Here's how the part is built. I have some questions about the finished solid (model axes, mm). Coordinates: 2 decimals unless noted, no trailing zeros. Loops run counter-clockwise (first coordinate to the right, second up) from the corner with the lowest first, then second, coordinate; pieces in that order, holes last. Notation, with made-up numbers: (-38.75, 79.5) -> (-9.75, 79.5) arc R6 ccw to (-9.75, 87.5) -> close; hole circle Ø2 at (4, -17). An arc over 180 degrees is marked (long way). Answer as a JSON object with one key per item and string values. Group by question number.
1) I want a section at B-B (x = -19.05). Write out the boundary of the cut face in (y, z), then the cut area to 3 significant figures.
2) I need wall thicknesses on probe 1 along Y at (x, z) = (-253, 1.5); probe 2 along X at (y, z) = (103, 1.5); probe 3 along X at (y, z) = (127.5, 3.75). Which ranges of each line are inside material? Lowest first, please. Write a range as [from, to].
3) I'm going to push flat-ended pins straight in: pin 1 (1.5 mm diameter, centred on y = 40.5, z = 4, fed in from -X); pin 2 (4 mm diameter, centred on x = -107, z = 1.5, fed in from -Y); pin 3 (3 mm diameter, centred on x = -216.5, z = 4, fed in from -Y). Where does each tip first touch, or does it pass through?
4) I want a section at D-D (y = 36). Write out the boundary of the cut face in (x, z), then the cut area to 3 significant figures.
5) I want a section at C-C (x = -192.5). Write out the boundary of the cut face in (y, z).
6) I want a section at A-A (y = 143). Write out the boundary of the cut face in (x, z).
```python
from build123d import *

# Parameters (mm, degrees)
SKETCH2_R               = 28.575
SKETCH2_R_2             = 3.2639
SKETCH2_R_3             = 52.3875
BOSS_EXTRUDE1_DEPTH     = 7.62
CUT_EXTRUDE1_DEPTH      = 369.573342704
CUT_EXTRUDE1_DEPTH_BACK = 369.573342704
SKETCH3_R               = 4.15
SKETCH3_R_2             = 2.5
CUT_EXTRUDE2_DEPTH      = 369.573342704
CUT_EXTRUDE2_DEPTH_BACK = 369.573342704


with BuildPart() as part:
    # Sketch2 → Boss-Extrude1 (new body)
    with BuildSketch(Plane.XY):
        with BuildLine():
            Line((-308.866129262, 91.710399516), (-215.926365234, 14.107506231))
            ThreePointArc((-215.926365234, 14.107506231), (-212.572921228, 12.657721799), (-208.970475069, 13.265869211))
            Line((-208.970475069, 13.265869211), (-134.814952137, 49.535152614))
            ThreePointArc((-134.814952137, 49.535152614), (-114.3, 46.0375), (-93.785047863, 49.535152614))
            Line((-93.785047863, 49.535152614), (-21.949808906, 13.301039962))
            ThreePointArc((-21.949808906, 13.301039962), (-14.699565425, 14.303090245), (-13.070560605, 21.438668609))
            Line((-13.070560605, 21.438668609), (-56.805390428, 130.917967399))
            ThreePointArc((-56.805390428, 130.917967399), (-79.09759936, 158.880822155), (-113.13445351, 169.85152791))
            Line((-113.13445351, 169.85152791), (-257.123397092, 172.562701825))
            ThreePointArc((-257.123397092, 172.562701825), (-258.950279318, 171.836030325), (-259.711214384, 170.023151962))
            Line((-259.711214384, 170.023151962), (-259.711214384, 163.648011794))
            ThreePointArc((-259.711214384, 163.648011794), (-266.061214384, 157.298011794), (-272.411214384, 163.648011794))
            Line((-272.411214384, 163.648011794), (-272.411214384, 170.357932335))
            ThreePointArc((-272.411214384, 170.357932335), (-273.138336021, 172.136997269), (-274.903397092, 172.897482198))
            Line((-274.903397092, 172.897482198), (-278.534507017, 172.96585252))
            ThreePointArc((-278.534507017, 172.96585252), (-281.325275441, 172.933669465), (-284.108948518, 172.732203969))
            ThreePointArc((-284.108948518, 172.732203969), (-285.734576401, 171.907148337), (-286.388785616, 170.205562866))
            Line((-286.388785616, 170.205562866), (-286.388785616, 163.648011794))
            ThreePointArc((-286.388785616, 163.648011794), (-292.738785616, 157.298011794), (-299.088785616, 163.648011794))
            Line((-299.088785616, 163.648011794), (-299.088785616, 164.31478857))
            ThreePointArc((-299.088785616, 164.31478857), (-300.373839326, 166.523115948), (-302.928714599, 166.496939949))
            ThreePointArc((-302.928714599, 166.496939949), (-325.229794091, 130.638495508), (-308.866129262, 91.710399516))
        make_face()
        with Locations(Location((-279.4, 127, 0), (0, 0, 180))):
            Circle(SKETCH2_R, mode=Mode.SUBTRACT)
        with Locations(Location((-19.05, 19.05, 0), (0, 0, 180))):
            Circle(SKETCH2_R_2, mode=Mode.SUBTRACT)
        with Locations(Location((-211.799479175, 19.05, 0), (0, 0, 180))):
            Circle(SKETCH2_R_2, mode=Mode.SUBTRACT)
        with Locations(Location((-114.3, 107.95, 0), (0, 0, 180))):
            Circle(SKETCH2_R_3, mode=Mode.SUBTRACT)
    extrude(amount=BOSS_EXTRUDE1_DEPTH)

    # Sketch3 → Cut-Extrude1 (cut, two sides: drawn at the far end of the back side and taken through both)
    with BuildSketch(Plane.XY.offset(7.62).offset(-CUT_EXTRUDE1_DEPTH_BACK)):
        with Locations((-279.4, 166.00043)):
            Circle(SKETCH3_R)
        with Locations((-254.746524018, 156.380868571)):
            Circle(SKETCH3_R)
        with Locations((-242.044200635, 133.164908097)):
            Circle(SKETCH3_R)
        with Locations((-247.236588134, 107.215554499)):
            Circle(SKETCH3_R)
        with Locations((-267.894110695, 90.674798722)):
            Circle(SKETCH3_R)
        with Locations((-294.35088393, 91.282244222)):
            Circle(SKETCH3_R)
        with Locations((-314.227489609, 108.753660501)):
            Circle(SKETCH3_R)
        with Locations((-318.223443029, 134.913977707)):
            Circle(SKETCH3_R)
        with Locations((-304.468993176, 157.522492681)):
            Circle(SKETCH3_R)
        with Locations((-114.3, 165.1)):
            Circle(SKETCH3_R_2)
        with Locations((-80.708072831, 154.185321229)):
            Circle(SKETCH3_R_2)
        with Locations((-59.947120094, 125.610321229)):
            Circle(SKETCH3_R_2)
        with Locations((-59.947120094, 90.289678771)):
            Circle(SKETCH3_R_2)
        with Locations((-80.708072831, 61.714678771)):
            Circle(SKETCH3_R_2)
        with Locations((-114.3, 50.8)):
            Circle(SKETCH3_R_2)
        with Locations((-147.891927169, 61.714678771)):
            Circle(SKETCH3_R_2)
        with Locations((-168.652879906, 90.289678771)):
            Circle(SKETCH3_R_2)
        with Locations((-168.652879906, 125.610321229)):
            Circle(SKETCH3_R_2)
        with Locations((-147.891927169, 154.185321229)):
            Circle(SKETCH3_R_2)
    extrude(amount=CUT_EXTRUDE1_DEPTH + CUT_EXTRUDE1_DEPTH_BACK, mode=Mode.SUBTRACT)

    # Sketch4 → Cut-Extrude2 (cut, two sides: drawn at the far end of the back side and taken through both)
    with BuildSketch(Plane.XY.offset(7.62).offset(-CUT_EXTRUDE2_DEPTH_BACK)):
        with BuildLine():
            Line((-278.862624236, 74.930604639), (-219.018129111, 24.961616472))
            ThreePointArc((-219.018129111, 24.961616472), (-217.07692299, 24.16262829), (-215.028330647, 24.620812453))
            ThreePointArc((-215.028330647, 24.620812453), (-211.026037121, 25.442278201), (-207.335161059, 23.689967346))
            ThreePointArc((-207.335161059, 23.689967346), (-205.454963796, 22.756414152), (-203.379217054, 23.069365873))
            Line((-203.379217054, 23.069365873), (-148.393096208, 49.962941986))
            ThreePointArc((-148.393096208, 49.962941986), (-146.441473652, 52.888826728), (-148.025123052, 56.029158988))
            ThreePointArc((-148.025123052, 56.029158988), (-167.199986736, 75.782484405), (-175.915777896, 101.895780766))
            ThreePointArc((-175.915777896, 101.895780766), (-177.021567584, 104.119565425), (-179.32579095, 105.046141768))
            Line((-179.32579095, 105.046141768), (-236.289123771, 106.118706774))
            ThreePointArc((-236.289123771, 106.118706774), (-238.085307811, 105.660495116), (-239.394002214, 104.347653165))
            ThreePointArc((-239.394002214, 104.347653165), (-255.140570758, 87.947615069), (-276.820157686, 81.098441316))
            ThreePointArc((-276.820157686, 81.098441316), (-279.939618833, 78.709346862), (-278.862624236, 74.930604639))
        make_face()
        with BuildLine():
            Line((-48.019318761, 91.807143198), (-22.303873454, 27.434904147))
            ThreePointArc((-22.303873454, 27.434904147), (-23.187455951, 23.564521405), (-27.120033775, 23.021003007))
            Line((-27.120033775, 23.021003007), (-80.387932313, 49.889641079))
            ThreePointArc((-80.387932313, 49.889641079), (-82.302626367, 52.822384958), (-80.709884678, 55.941714036))
            ThreePointArc((-80.709884678, 55.941714036), (-64.405072396, 71.294115674), (-54.62867895, 91.442695545))
            ThreePointArc((-54.62867895, 91.442695545), (-51.454892751, 93.998716793), (-48.019318761, 91.807143198))
        make_face()
        with BuildLine():
            Line((-243.589870481, 164.686527829), (-154.467376545, 163.008436618))
            ThreePointArc((-154.467376545, 163.008436618), (-151.219977886, 160.621367905), (-152.384754551, 156.763001619))
            ThreePointArc((-152.384754551, 156.763001619), (-168.119955828, 138.553431359), (-175.723033577, 115.719723447))
            ThreePointArc((-175.723033577, 115.719723447), (-176.903269485, 113.516440978), (-179.253671427, 112.666134477))
            Line((-179.253671427, 112.666134477), (-230.993471474, 113.640345363))
            ThreePointArc((-230.993471474, 113.640345363), (-233.653099209, 114.948221132), (-234.350027257, 117.828924174))
            ThreePointArc((-234.350027257, 117.828924174), (-235.231792854, 139.758454197), (-246.179291838, 158.780390577))
            ThreePointArc((-246.179291838, 158.780390577), (-246.854206706, 162.596999998), (-243.589870481, 164.686527829))
        make_face()
    extrude(amount=CUT_EXTRUDE2_DEPTH + CUT_EXTRUDE2_DEPTH_BACK, mode=Mode.SUBTRACT)


solid = part.part
```
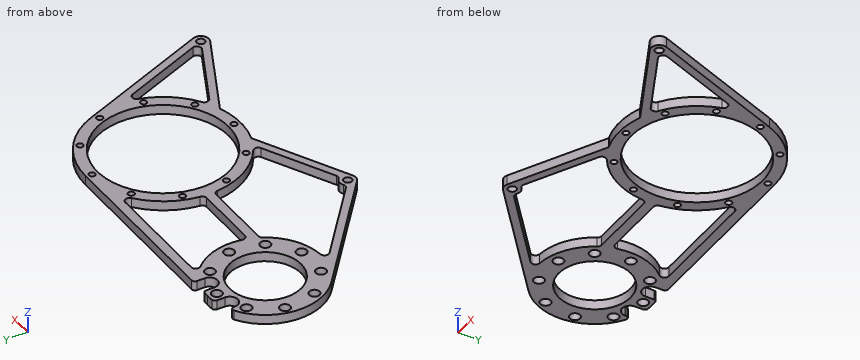
Determined:
{
 "1": {"outline": "(12.61, 0) -> (15.79, 0) -> (15.79, 7.62) -> (12.61, 7.62) -> close; (22.31, 0) -> (36.41, 0) -> (36.41, 7.62) -> (22.31, 7.62) -> close", "area": "132 mm^2"},
 "2": {"probe 1": "[45.06, 53.34], [89.36, 116.07], [137.93, 152.62], [160.15, 172.49]", "probe 2": "[-318.61, -294.91], [-263.89, -240.19], [-176.21, -166.45], [-62.15, -45.65]", "probe 3": "[-325.37, -307.97], [-250.83, -233.43], [-173.04, -170.29], [-167.02, -162.9], [-65.7, -61.58], [-58.31, -55.44]"},
 "3": {"pin 1": "x = -248.43", "pin 2": "y = 46.26", "pin 3": "y = 13.46"},
 "4": {"outline": "(-242.15, 0) -> (-232.24, 0) -> (-232.24, 7.62) -> (-242.15, 7.62) -> close; (-176.94, 0) -> (-162.49, 0) -> (-162.49, 7.62) -> (-176.94, 7.62) -> close; (-66.95, 0) -> (-52.85, 0) -> (-52.85, 7.62) -> (-66.95, 7.62) -> close; (-25.73, 0) -> (-18.89, 0) -> (-18.89, 7.62) -> (-25.73, 7.62) -> close", "area": "345 mm^2"},
 "5": {"outline": "(21.32, 0) -> (28.39, 0) -> (28.39, 7.62) -> (21.32, 7.62) -> close; (105.29, 0) -> (112.92, 0) -> (112.92, 7.62) -> (105.29, 7.62) -> close; (163.72, 0) -> (171.35, 0) -> (171.35, 7.62) -> (163.72, 7.62) -> close"},
 "6": {"outline": "(-322.5, 0) -> (-303.08, 0) -> (-303.08, 7.62) -> (-322.5, 7.62) -> close; (-255.72, 0) -> (-236.3, 0) -> (-236.3, 7.62) -> (-255.72, 7.62) -> close; (-165.34, 0) -> (-153.24, 0) -> (-153.24, 7.62) -> (-165.34, 7.62) -> close; (-75.36, 0) -> (-63.26, 0) -> (-63.26, 7.62) -> (-75.36, 7.62) -> close"}
}
